The listing builds one solid part. Answer for the finished solid, in the listing's coordinates (mm). Give positions to 0.01 mm unless a question says otherwise; leave off trailing zeros. Write each loop counter-clockwise with the first axis right and the second up, starting at its lowest first coordinate (ties: lowest second). Pieces come first, ordered by that corner, then holes. Notation, with made-up numbers: (53.25, -29) - (94.25, -29) arc R34 ccw to (94.25, 7) - close; hole circle Ø10 at (39.5, 44). An arc over 180 degrees is marked (long way). Return JSON: item names as keys, results as strings.
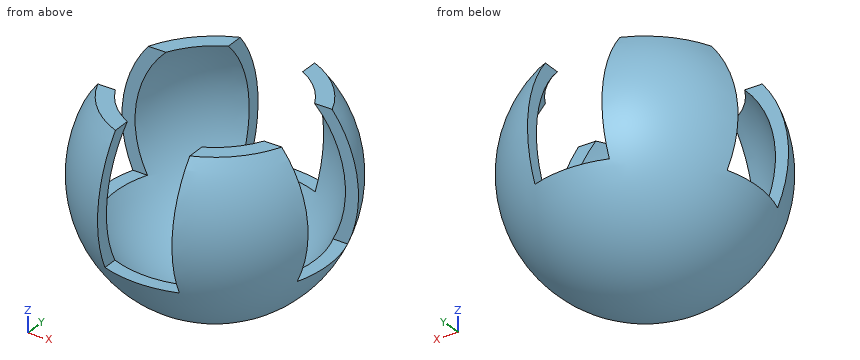
from build123d import *

# Parameters (mm, degrees)
BOX004_W               = 6
BOX004_H               = 20
BOX004_DEPTH           = 20
BOX004_PLACEMENT_ANGLE = 90
BOX003_W               = 6
BOX003_H               = 20
BOX003_DEPTH           = 20
BOX001_W               = 20
BOX001_H               = 20
BOX001_DEPTH           = 20
THICKNESS_T            = -1


with BuildPart() as cube004:
    # Box004 → Box004 (new body)
    with BuildSketch(Plane.XY):
        with Locations((3, 10)):
            Rectangle(BOX004_W, BOX004_H)
    extrude(amount=BOX004_DEPTH)


with BuildPart() as cube004_1:
    # Box004 placement: moved
    add(cube004.part.moved(Location((10, -3, -4))).rotate(Axis((10, -3, -4), (0, 0, 1)), BOX004_PLACEMENT_ANGLE))


with BuildPart() as fusion:
    # Box003 → Box003 (new body)
    with BuildSketch(Plane(origin=(-3, -10, -4), x_dir=(1, 0, 0), z_dir=(0, 0, 1))):
        with Locations((3, 10)):
            Rectangle(BOX003_W, BOX003_H)
    extrude(amount=BOX003_DEPTH)

    # Fusion: union Cube004
    add(cube004_1.part)


with BuildPart() as cube001:
    # Box001 → Box001 (new body)
    with BuildSketch(Plane(origin=(-10, -10, 6), x_dir=(1, 0, 0), z_dir=(0, 0, 1))):
        with Locations((10, 10)):
            Rectangle(BOX001_W, BOX001_H)
    extrude(amount=BOX001_DEPTH)


with BuildPart() as cut001:
    # Sphere → Sphere (revolve)
    with BuildSketch(Plane.XZ):
        with BuildLine():
            ThreePointArc((0, -10), (10, 0), (0, 10))
            Line((0, 10), (0, -10))
        make_face()
    revolve(axis=Axis((0, 0, 0), (0, 0, 1)))

    # Cut: cut Cube001
    add(cube001.part, mode=Mode.SUBTRACT)

    # Thickness
    thickness_openings = [cut001.faces().sort_by_distance(p)[0] for p in [
        (0, 0, 6),
    ]]
    offset(amount=THICKNESS_T, openings=thickness_openings, kind=Kind.INTERSECTION)

    # Cut001: cut Fusion
    add(fusion.part, mode=Mode.SUBTRACT)


solid = cut001.part
Item 1: A cutting plane is placed at B-B on x = 7.75. Determine the outline of the cut face in (y, z).
Answer below:
{"outline": "(-3, -4) - (-3, -3.46) arc R4.58 cw to (-3, 3.46) - (-3, 5.56) arc R6.32 ccw (long way) to (3, 5.56) - (3, 3.46) arc R4.58 cw to (3, -3.46) - (3, -4) - (2.22, -4) arc R4.58 cw to (-2.22, -4) - close"}
Item 2: A cutting plane is placed at C-C on z = -3.5. Determine the outline of the cut face in (x, y) (1 decimal).
Answer below:
{"outline": "(-8.9, -3) arc R9.4 ccw to (-3, -8.9) - (-3, -7.7) arc R8.3 cw to (-7.7, -3) - close; (-8.9, 3) - (-7.7, 3) arc R8.3 cw to (-3, 7.7) - (-3, 8.9) arc R9.4 ccw to start; (3, -8.9) arc R9.4 ccw to (8.9, -3) - (7.7, -3) arc R8.3 cw to (3, -7.7) - close; (3, 7.7) arc R8.3 cw to (7.7, 3) - (8.9, 3) arc R9.4 ccw to (3, 8.9) - close"}
Item 3: A cutting plane is placed at D-D on y = -0.5. Determine the outline of the cut face in (x, z).
Answer below:
{"outline": "(-9.15, -4) arc R9.99 ccw to (9.15, -4) - (8.05, -4) arc R8.99 cw to (-8.05, -4) - close"}
Item 4: A cutting plane is placed at A-A on z = -0.5. Determine the outline of the cut face in (x, y), then the cut area to 3 significant figures.
Answer below:
{"outline": "(-9.53, -3) arc R9.99 ccw to (-3, -9.53) - (-3, -8.47) arc R8.99 cw to (-8.47, -3) - close; (-9.53, 3) - (-8.47, 3) arc R8.99 cw to (-3, 8.47) - (-3, 9.53) arc R9.99 ccw to start; (3, -9.53) arc R9.99 ccw to (9.53, -3) - (8.47, -3) arc R8.99 cw to (3, -8.47) - close; (3, 8.47) arc R8.99 cw to (8.47, 3) - (9.53, 3) arc R9.99 ccw to (3, 9.53) - close", "area": "35.2 mm²"}
Item 5: Consider L1, parallel to Y at x = -7, z = -3.5; L2, parallel to X at y = -4, z = 2.5; L3, parallel to X at y = -3.5, z = 0.25. Determine where each line is inside the solid, lowest interval first.
Answer below:
{"L1": "y = -6.22 to -4.44, 4.44 to 6.22", "L2": "x = -8.82 to -7.66, 7.66 to 8.82", "L3": "x = -9.36 to -8.29, 8.29 to 9.36"}
Item 6: Flat-ended cylindrical pins translate along their axes: P1, Ø3, axis at y = 7.5, z = 2.5, coming from the +X side; P2, Ø4, axis at y = -8.5, z = 0, coming from the -X side; P3, Ø4, axis at y = 7.5, z = 0, coming from the -X side. Find the tip coordinate at first contact, or state that the pin passes through.
Answer below:
{"P1": "stops at x = 7.68", "P2": "stops at x = -7.6", "P3": "stops at x = -8.35"}
